from build123d import *

# Parameters (mm, degrees)
F1_DEPTH     = 101.6
F2_T1_DEPTH  = 101.6
F2_T3_DEPTH  = 118.1792407144
F2_T5_DEPTH  = 29.422869264
F2_T7_DEPTH  = 60.4590704492
F2_T10_ANGLE = 73.6909129446
F2_T12_ANGLE = 73.6909129446


# Not quite as in the source:
# - a fillet or chamfer that OpenCascade refuses, or shapes differently, is made with other operations: its cross-section is extruded or revolved along the edge and cut away or added


with BuildPart() as f1:
    # F0 (on Right) → F1 (new body)
    with BuildSketch(Plane.YZ):
        Polygon((15.3971137479, -57.599131723), (15.3971137479, -53.6149479449), (-34.0936109424, -53.6149479449), (13.9307221398, -40.600720793), (-33.1771150231, -40.600720793), (21.9958759844, -34.3685559928), (21.9958759844, 0), (11.3645363599, -4.6741236001), (11.3645363599, -25.2036079764), (-38.1261855364, -39.6842285991), (-36.6007449852, -44.8977588791), (0, -42.4337126315), (-39.1800553827, -53.0512081353), (-37.9476028562, -57.599131723), align=None)
    extrude(amount=F1_DEPTH)

    # F2: fillet of radius 5.08 on 6 edges, made by hand

    # F2_s2 → F2_t1 (join)
    with BuildSketch(Plane.YZ):
        with BuildLine():
            ThreePointArc((11.3645363599, -21.3969928641), (10.3498362027, -24.44325897), (7.7110965222, -26.2725775576))
            Line((7.7110965222, -26.2725775576), (11.3645363599, -25.2036079764))
            Line((11.3645363599, -25.2036079764), (11.3645363599, -21.3969928641))
        make_face()
    extrude(amount=F2_T1_DEPTH)

    # F2_s4 → F2_t3 (cut)
    with BuildSketch(Plane.YZ.offset(-8.2896203572)):
        with BuildLine():
            ThreePointArc((14.3999677165, -3.3395804625), (12.1905494824, -5.2132838517), (11.3645363599, -7.989971743))
            Line((11.3645363599, -7.989971743), (11.3645363599, -4.6741236001))
            Line((11.3645363599, -4.6741236001), (14.3999677165, -3.3395804625))
        make_face()
    extrude(amount=F2_T3_DEPTH, mode=Mode.SUBTRACT)

    # F2_s6 → F2_t5 (cut)
    with BuildSketch(Plane.XY.offset(-21.3969928641)):
        with BuildLine():
            ThreePointArc((0, 16.4445363599), (1.4878975516, 12.8524339115), (5.08, 11.3645363599))
            Line((5.08, 11.3645363599), (0, 11.3645363599))
            Line((0, 11.3645363599), (0, 16.4445363599))
        make_face()
        with BuildLine():
            ThreePointArc((101.6, 16.4445363599), (100.1121024484, 12.8524339115), (96.52, 11.3645363599))
            Line((96.52, 11.3645363599), (101.6, 11.3645363599))
            Line((101.6, 11.3645363599), (101.6, 16.4445363599))
        make_face()
    extrude(amount=F2_T5_DEPTH, mode=Mode.SUBTRACT)

    # F2_s8 → F2_t7 (cut)
    with BuildSketch(Plane(origin=(0, 0.0220464736, 0.0064506358), x_dir=(1, 0, 0), z_dir=(0, -0.9597607664, -0.2808189296))):
        with BuildLine():
            ThreePointArc((0, -32.4608110442), (1.4878975516, -28.8687085958), (5.08, -27.3808110442))
            Line((5.08, -27.3808110442), (0, -27.3808110442))
            Line((0, -27.3808110442), (0, -32.4608110442))
        make_face()
        with BuildLine():
            ThreePointArc((101.6, -32.4608110442), (100.1121024484, -28.8687085958), (96.52, -27.3808110442))
            Line((96.52, -27.3808110442), (101.6, -27.3808110442))
            Line((101.6, -27.3808110442), (101.6, -32.4608110442))
        make_face()
    extrude(amount=F2_T7_DEPTH, mode=Mode.SUBTRACT)

    # F2_s9 → F2_t10 (revolve, cut)
    with BuildSketch(Plane.XY.offset(-21.3969928641)):
        with BuildLine():
            ThreePointArc((101.6, 16.4445363599), (100.1121024484, 12.8524339115), (96.52, 11.3645363599))
            Line((96.52, 11.3645363599), (101.6, 11.3645363599))
            Line((101.6, 11.3645363599), (101.6, 16.4445363599))
        make_face()
    revolve(axis=Axis((101.6, 6.2845363599, -21.3969928641), (-1, 0, 0)), revolution_arc=F2_T10_ANGLE, mode=Mode.SUBTRACT)

    # F2_s11 → F2_t12 (revolve, cut)
    with BuildSketch(Plane.XY.offset(-21.3969928641)):
        with BuildLine():
            ThreePointArc((0, 16.4445363599), (1.4878975516, 12.8524339115), (5.08, 11.3645363599))
            Line((5.08, 11.3645363599), (0, 11.3645363599))
            Line((0, 11.3645363599), (0, 16.4445363599))
        make_face()
    revolve(axis=Axis((0, 6.2845363599, -21.3969928641), (-1, 0, 0)), revolution_arc=F2_T12_ANGLE, mode=Mode.SUBTRACT)


solid = f1.part
The listing builds one solid part. Answer for the finished solid, in the listing's coordinates (mm). A direction names the side the tool comes from. Coordinates: 2 decimals unless noted, no trailing zeros. Write each loop counter-clockwise with the first axis right and the second up, starting at its lowest first coordinate (ties: lowest second). Pieces come first, ordered by that corner, then holes. Notation, with made-up numbers: (30.5, 78.25) -> (83.5, 78.25) arc R22 ccw to (83.5, 95.25) -> close; hole circle Ø11 at (40, 73.5). An arc over 180 degrees is marked (long way). One line per question, with ' | ' between items.
1. Which of the six approach directions +Z, -Z, +X, -X, +Y, -Y give full straight-line access (tool end or side, diameter ignored) to faces 1 (the flat face through (50.089, -37.374, -42.254)), 2 (the flat face through (50, 15.397, -56)), 3 (the flat face through (50, -9, -53.615)), 4 (the cylindrical face through (100.15, 12.89, -12.05)), 5 (the cylindrical face through (1.45, 12.89, -12.05))?
Verdict:
face 1: +X, -X, -Y | face 2: -Z, +X, -X, +Y | face 3: +X, -X, +Y | face 4: +Z, +X, -Y | face 5: +Z, -X, -Y
2. For a pull along Z with two mould halves and no side action, classify faces 6 (the flat face through (50, 21.996, -17)), 7 (the flat face through (50.09, -5.98, -37.53)), 8 (the flat face through (50.089, 18.251, -1.646)) as released by +Z, released by -Z, zero draft, split by the parting line, or undercut.
Verdict:
face 6: zero draft | face 7: undercut | face 8: released by +Z
3. Section A-A (z = -12) is taken. Determine the outline of the cut face in (x, y), and give its area (3 significant figures).
Verdict:
outline: (0, 16.44) arc R5.08 ccw to (5.08, 11.36) -> (96.52, 11.36) arc R5.08 ccw to (101.6, 16.44) -> (101.6, 22) -> (0, 22) -> close | area: 1,070 mm^2
4. Given pin 1 Ø6 at (x, y) = (76, 6) entering from +Z; pin 2 Ø24.5 at (x, y) = (61.5, -15.5) entering from +Z; pin 3 Ø6.5 at (x, z) = (67, -12.5) entering from -Y, each flat-ended and moving along its own axis, determine where each tip first touches the part or whether it passes through.
Verdict:
pin 1: stops at z = -25.69 | pin 2: stops at z = -29.48 | pin 3: stops at y = 11.36
5. Section B-B (x = 55) is taken. Determine the outline of the cut face in (y, z).
Verdict:
outline: (-39.18, -53.05) -> (-37.95, -57.6) -> (15.4, -57.6) -> (15.4, -53.61) -> (-34.09, -53.61) -> (13.93, -40.6) -> (-33.18, -40.6) -> (22, -34.37) -> (22, 0) -> (14.4, -3.34) arc R5.08 ccw to (11.36, -7.99) -> (11.36, -21.4) arc R5.08 cw to (7.71, -26.27) -> (-38.13, -39.68) -> (-36.6, -44.9) -> (0, -42.43) -> close
6. Section C-C (y = -7) is taken. State how many separate pieces and enclosed holes the cut face has, and give its area (3 significant figures).
Verdict:
separate pieces: 4 | enclosed holes: 0 | area: 1,540 mm^2
7. Straight lines are drawn through the part: line 1 (Z direction, x = 70, y = 5); line 2 (Z direction, x = 83, y = -33.5); line 3 (Z direction, x = 22, y = -11.5). For each, find the intervals that lie inside material, in ascending order.
Verdict:
line 1: z = -57.6 to -53.61, -43.02 to -40.6, -36.29 to -27.07 | line 2: z = -57.6 to -53.61, -53.45 to -51.51, -44.69 to -38.33 | line 3: z = -57.6 to -53.61, -47.49 to -45.55, -43.21 to -40.6, -38.15 to -31.89
